Design review of the part built by this model. Coordinates are the model's own, in mm. Face numbers are marked on the shaded views. A direction names the side the tool comes from. Coordinates: 2 decimals unless noted, no trailing zeros. Write each loop counter-clockwise with the first axis right and the second up, starting at its lowest first coordinate (ties: lowest second). Pieces come first, ordered by that corner, then holes. Notation, with made-up numbers: M -3.75,53 L 32.25,53 A17 cw 32.25,74 Z; hole C 52,-27.75 d1. An arc over 180 degrees is marked long. One line per question, with ' | ' between items.
from build123d import *

# Parameters (mm, degrees)
BOSS_EXTRUDE1_DEPTH = 208
SHELL1_T            = -1.33


with BuildPart() as part:
    # Sketch1 → Boss-Extrude1 (new body)
    with BuildSketch(Plane.XY):
        with BuildLine():
            Line((-33, -17.25), (33, -17.25))
            ThreePointArc((33, -17.25), (34.767766953, -16.517766953), (35.5, -14.75))
            Line((35.5, -14.75), (35.5, 14.75))
            ThreePointArc((35.5, 14.75), (34.767766953, 16.517766953), (33, 17.25))
            Line((33, 17.25), (-33, 17.25))
            ThreePointArc((-33, 17.25), (-34.767766953, 16.517766953), (-35.5, 14.75))
            Line((-35.5, 14.75), (-35.5, -14.75))
            ThreePointArc((-35.5, -14.75), (-34.767766953, -16.517766953), (-33, -17.25))
        make_face()
    extrude(amount=-BOSS_EXTRUDE1_DEPTH)

    # Shell1
    shell1_openings = [part.faces().sort_by_distance(p)[0] for p in [
        (0, 0, -208),
        (0, 0, 0),
    ]]
    offset(amount=SHELL1_T, openings=shell1_openings, kind=Kind.INTERSECTION)


solid = part.part
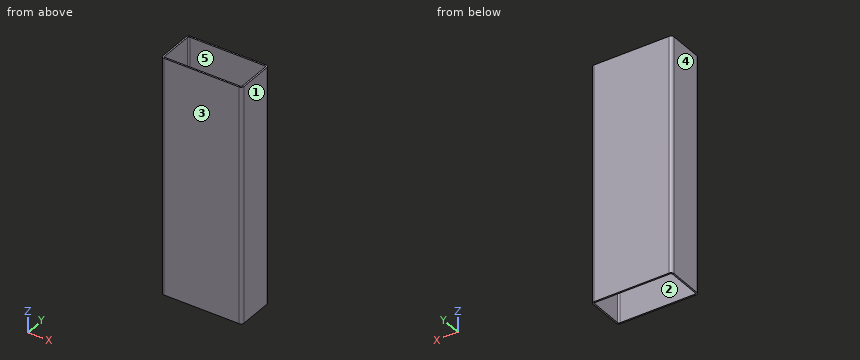
1. Insertion check: pin 1 Ø3 at (x, y) = (-21, -13) entering from -Z. The pin has a flat end and moves straight along its axis. Give the tip position at first contact, or say it passes through.
Answer sheet:
pin 1: through
2. Take a section at B-B (y = -6.5). Write out the cut boundary in (x, z).
Answer sheet:
outline: M -35.5,-208 L -34.17,-208 L -34.17,0 L -35.5,0 Z; M 34.17,-208 L 35.5,-208 L 35.5,0 L 34.17,0 Z
3. Take a section at C-C (z = -110). Write out the cut boundary in (x, y), then the cut area to 3 significant figures.
Answer sheet:
outline: M -35.5,-14.75 A2.5 ccw -33,-17.25 L 33,-17.25 A2.5 ccw 35.5,-14.75 L 35.5,14.75 A2.5 ccw 33,17.25 L -33,17.25 A2.5 ccw -35.5,14.75 Z; hole M -34.17,-14.75 A1.17 ccw -33,-15.92 L 33,-15.92 A1.17 ccw 34.17,-14.75 L 34.17,14.75 A1.17 ccw 33,15.92 L -33,15.92 A1.17 ccw -34.17,14.75 Z | area: 269 mm^2
4. To check wall thickness, follow line 1 along Y through (x, z) = (-14.5, -106); line 2 along X through (y, z) = (1, -10). State the ranges of each line that lie inside material, in increasing order. Write a range as [from, to].
Answer sheet:
line 1: [-17.25, -15.92], [15.92, 17.25] | line 2: [-35.5, -34.17], [34.17, 35.5]
5. Take a section at A-A (x = 0). Write out the cut boundary in (y, z).
Answer sheet:
outline: M -17.25,-208 L -15.92,-208 L -15.92,0 L -17.25,0 Z; M 15.92,-208 L 17.25,-208 L 17.25,0 L 15.92,0 Z
6. Draft analysis for pull direction X (two halves, no side actions). For the marked faces 1, 2 and 3, state which applies: pulls with the +X half, pulls with the -X half, needs draft (parallel to the pull), parting line crosses it, or undercut.
Answer sheet:
face 1: pulls with the +X half | face 2: undercut | face 3: needs draft
7. Tool access review of the marked faces 4 and 5: name each direction out of +Z, -Z, +X, -X, +Y, -Y from which nothing blocks a thin tool from reaching the whole face with its end or side.
Answer sheet:
face 4: +Z, -Z, -X, +Y, -Y | face 5: +Z, -Z
